Geometry check sheet. Reference: the model listing, model coordinates, mm. A direction names the side the tool comes from. Give positions to 0.01 mm unless a question says otherwise; leave off trailing zeros. Loops run counter-clockwise (first coordinate to the right, second up) from the corner with the lowest first, then second, coordinate; pieces in that order, holes last.
```python
from build123d import *

# Parameters (mm, degrees)
SKETCH_1_R          = 2
SKETCH_1_R_2        = 1.25
EXTRUDE_1_DEPTH     = 2
SKETCH_3_W          = 33
SKETCH_3_H          = 6
SKETCH_3_H_2        = 58
SKETCH_3_W_2        = 34.5
SKETCH_3_H_3        = 49.5
CUT_EXTRUDE_2_DEPTH = 130.341601969
SKETCH_2_R          = 0.75
CUT_EXTRUDE_1_DEPTH = 130.341601969
EXTRUDE_1_2_DEPTH   = 2
FILLET_1_R          = 1
FILLET_2_R          = 2


with BuildPart() as part:
    # 草图1 → Extrude 1 (new body)
    with BuildSketch(Plane(origin=(0, 0, 0), x_dir=(1, 0, 0), z_dir=(0, 1, 0))):
        Polygon((0, 0), (30, 0), (30, 2), (95, 2), (105, -8), (105, -72.5), (83, -72.5), (83, -75.5), (43, -75.5), (43, -72.5), (0, -72.5), align=None)
        with Locations(Location((7.5, -7.5, 0), (0, 0, 270))):
            Circle(SKETCH_1_R, mode=Mode.SUBTRACT)
        with Locations(Location((22.5, -7.5, 0), (0, 0, 270))):
            Circle(SKETCH_1_R, mode=Mode.SUBTRACT)
        with Locations(Location((42, -3.75, 0), (0, 0, 270))):
            Circle(SKETCH_1_R_2, mode=Mode.SUBTRACT)
        with Locations(Location((42, -66.75, 0), (0, 0, 270))):
            Circle(SKETCH_1_R_2, mode=Mode.SUBTRACT)
        with Locations(Location((84, -66.75, 0), (0, 0, 270))):
            Circle(SKETCH_1_R_2, mode=Mode.SUBTRACT)
        with Locations(Location((84, -3.75, 0), (0, 0, 270))):
            Circle(SKETCH_1_R_2, mode=Mode.SUBTRACT)
    extrude(amount=EXTRUDE_1_DEPTH)

    # 草图3 → 切除-拉伸2 (cut, through all)
    with BuildSketch(Plane(origin=(0, 2, 0), x_dir=(1, 0, 0), z_dir=(0, 1, 0))):
        with Locations((63, -5)):
            Rectangle(SKETCH_3_W, SKETCH_3_H)
        with Locations((63, -42)):
            Rectangle(SKETCH_3_W, SKETCH_3_H_2)
        with Locations((23.25, -37.75)):
            Rectangle(SKETCH_3_W_2, SKETCH_3_H_3)
        Polygon((93.686291501, -8), (99, -13.313708499), (99, -62.5), (85.5, -62.5), (85.5, -8), align=None)
    extrude(amount=-CUT_EXTRUDE_2_DEPTH, mode=Mode.SUBTRACT)

    # 草图2 → 切除-拉伸1 (cut, through all)
    with BuildSketch(Plane(origin=(0, 2, 0), x_dir=(1, 0, 0), z_dir=(0, 1, 0))):
        with Locations((42.25, -72.5)):
            Circle(SKETCH_2_R)
        with Locations((83.75, -72.5)):
            Circle(SKETCH_2_R)
    extrude(amount=-CUT_EXTRUDE_1_DEPTH, mode=Mode.SUBTRACT)

    # 草图4 → Extrude 1 2 (add)
    with BuildSketch(Plane(origin=(0, 2, 0), x_dir=(1, 0, 0), z_dir=(0, 1, 0))):
        Polygon((3.949004583, -14.429481654), (38.449004583, -63.929481654), (42.550995417, -61.070518346), (8.050995417, -11.570518346), align=None)
    extrude(amount=-EXTRUDE_1_2_DEPTH)

    # 圆角1
    fillet_1_edges = [part.edges().sort_by_distance(p)[0] for p in [
        (0, 1, 0),
        (83, 1, 75.5),
        (0, 1, 72.5),
        (43, 1, 75.5),
        (105, 1, 72.5),
        (30, 1, -2),
        (30, 1, 0),
        (105, 1, 8),
        (95, 1, -2),
        (46.5, 1, 71),
        (46.5, 1, 13),
        (79.5, 1, 13),
        (79.5, 1, 71),
        (46.5, 1, 8),
        (46.5, 1, 2),
        (79.5, 1, 2),
        (79.5, 1, 8),
        (99, 1, 62.5),
        (85.5, 1, 62.5),
        (85.5, 1, 8),
        (37.452699188, 1, 62.5),
        (40.5, 1, 58.127785791),
        (6, 1, 17.372214209),
        (9.047300812, 1, 13),
    ]]
    fillet(fillet_1_edges, radius=FILLET_1_R - 0.0001)  # a hair under: the kernel refuses the full size

    # 圆角2
    fillet_2_edges = [part.edges().sort_by_distance(p)[0] for p in [
        (93.686291501, 1, 8),
        (99, 1, 13.313708499),
        (6, 1, 62.5),
        (40.5, 1, 13),
    ]]
    fillet(fillet_2_edges, radius=FILLET_2_R)


solid = part.part
```
1) Sectioned sample at C-C on x = 22.5. Enter the section's corners in (y, z), plus the area to 3 significant figures.
2) Sectioned sample at D-D on y = 0.55. Count the separate pieces of the cut face and the enclosed holes in it, plus the area to 3 significant figures.
3) Depth check by flat-ended pin: P1, Ø3, axis at x = 84, z = 66.75, coming from the -Y side; P2, Ø0.6, axis at x = 96.5, y = 0.5, coming from the +Z side. Enter the tip coordinate at first touch or a pass-through.
4) Tool access check on faces 5 (the flat face through (46.5, 1, 5)), 6 (the flat face through (62, 1, -2)). Record the directions out of +Z, -Z, +X, -X, +Y, -Y that give a thin tool (end or side, any length) a straight path to the whole face; none if there is none.
5) Mould release check, pull along X, two halves, no side actions. Record for faces 1 (the flat face through (22, 1, 72.5)), 2 (the flat face through (100, 1, 3)), 3 (the flat face through (25, 1, 13)), 4 (the cylindrical face through (39.93, 0.99, 13.6)): +X half, -X half, draft (parallel to the pull), parting line (faces both ways), or undercut.
6) Sectioned sample at B-B on z = 66.75. Enter the section's corners in (x, y), plus the area to 3 significant figures.
7) Scan lines: line 1 along X through (y, z) = (0.8, 66.75); line 2 along X through (y, z) = (1.05, 3.75); line 3 along Z through (x, y) = (84, 0.6). Record each from-to range of solid material in increasing order.
8) Sectioned sample at A-A on x = 68. Enter the section's corners in (y, z), plus the area to 3 significant figures.
Determined:
1. outline: (0, 0) - (2, 0) - (2, 5.5) - (0, 5.5) - close; (0, 9.5) - (2, 9.5) - (2, 13) - (0, 13) - close; (0, 32.3) - (2, 32.3) - (2, 41.05) - (0, 41.05) - close; (0, 62.5) - (2, 62.5) - (2, 72.5) - (0, 72.5) - close
1. area: 55.5 mm2
2. separate pieces: 1
2. enclosed holes: 11
2. area: 3,540 mm2
3. P1: stops at y = 0
3. P2: stops at z = 72.5
4. face 5: +Y, -Y
4. face 6: -Z, +X, -X, +Y, -Y
5. face 1: draft
5. face 2: +X half
5. face 3: undercut
5. face 4: undercut
6. outline: (0, 0) - (40.75, 0) - (40.75, 2) - (0, 2) - close; (43.25, 0) - (46.5, 0) - (46.5, 2) - (43.25, 2) - close; (79.5, 0) - (82.75, 0) - (82.75, 2) - (79.5, 2) - close; (85.25, 0) - (105, 0) - (105, 2) - (85.25, 2) - close
6. area: 134 mm2
7. line 1: x = 0 to 40.75, 43.25 to 46.5, 79.5 to 82.75, 85.25 to 105
7. line 2: x = 0 to 40.75, 43.25 to 46.5, 79.5 to 82.75, 85.25 to 100.75
7. line 3: z = -2 to 2.5, 5 to 65.5, 68 to 71.79
8. outline: (0, -2) - (2, -2) - (2, 2) - (0, 2) - close; (0, 8) - (2, 8) - (2, 13) - (0, 13) - close; (0, 71) - (2, 71) - (2, 75.5) - (0, 75.5) - close
8. area: 27.0 mm2
